Autodesk Inventor part; units mm, degrees
ref_plane "YZ Plane" through (0, 0, 0) normal (1, 0, 0) x (0, 1, 0)
ref_plane "XZ Plane" through (0, 0, 0) normal (0, 1, 0) x (-1, 0, 0)
ref_plane "XY Plane" through (0, 0, 0) normal (0, 0, 1) x (1, 0, 0)
sketch "Sketch1" plane through (0, 0, 0) normal (0, 0, 1) x (1, 0, 0)
  line L0 (0, 0) -> (620, 0)
  line L1 (620, 0) -> (620, 620)
  line L2 (620, 620) -> (0, 620)
  line L3 (0, 620) -> (0, 0)
  dimension "d0" = 620
  dimension "d1" = 620
extrude "Extrusion1" add sketch "Sketch1" along normal blind 10
sketch "Sketch2" plane through (0, 0, 10) normal (0, 0, 1) x (1, 0, 0)
  line L0 (193.5, 388) -> (406.5, 388)
  line L1 (406.5, 388) -> (406.5, 501)
  line L2 (406.5, 501) -> (193.5, 501)
  line L3 (193.5, 501) -> (193.5, 388)
  line L4 (0, 620) -> (0, 0)
  line L5 (620, 620) -> (0, 620)
  dimension "d4" = 213
  dimension "d5" = 113
  dimension "d6" = 193.5
  dimension "d7" = 119
extrude "Extrusion2" cut sketch "Sketch2" against normal through all
properties part number "Top Cover" material "ABS Plastic"
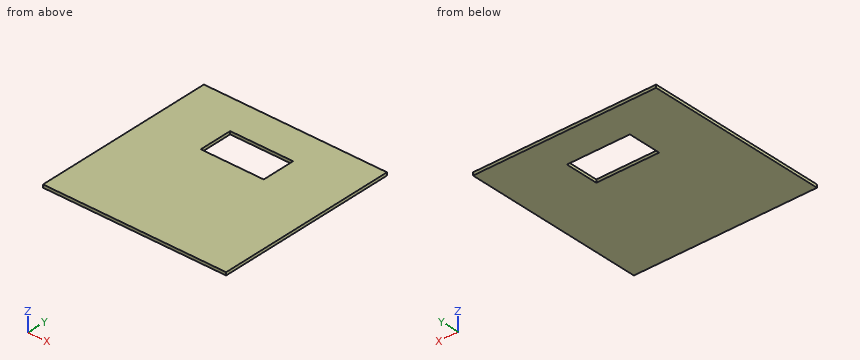
Could you check a few things on this model? Use its own coordinates, in mm. Round coordinates to 2 decimals unless told otherwise and drop trailing zeros. Write each loop counter-clockwise with the first axis right and the second up, starting at its lowest first coordinate (ties: lowest second). Pieces come first, ordered by that corner, then holes. Notation, with made-up numbers: (-35.5, 52) - (-1.5, 52) arc R21 cw to (-1.5, 65) - close; hole circle Ø9 at (76, -7.75). An arc over 180 degrees is marked (long way). Put each result on its own line as item: value. Start each with the question number.
(1) I want a section at B-B, the plane z = 4.5. Please give me the cut outline in (x, y).
(2) I need wall thicknesses on probe 1 along Y at (x, z) = (264.5, 6); probe 2 along X at (y, z) = (419.5, 3.5). Which ranges of each line are inside material? Lowest first, please.
(3) I want a section at C-C, the plane x = 332. Please give me the cut outline in (y, z), plus the area to 3 significant figures.
(4) I want a section at A-A, the plane y = 460. Please give me the cut outline in (x, z), plus the area to 3 significant figures.
Here are the results:
1. outline: (0, 0) - (620, 0) - (620, 620) - (0, 620) - close; hole (193.5, 388) - (406.5, 388) - (406.5, 501) - (193.5, 501) - close
2. probe 1: y = 0 to 388, 501 to 620
2. probe 2: x = 0 to 193.5, 406.5 to 620
3. outline: (0, 0) - (388, 0) - (388, 10) - (0, 10) - close; (501, 0) - (620, 0) - (620, 10) - (501, 10) - close
3. area: 5,070 mm^2
4. outline: (0, 0) - (193.5, 0) - (193.5, 10) - (0, 10) - close; (406.5, 0) - (620, 0) - (620, 10) - (406.5, 10) - close
4. area: 4,070 mm^2
